Design review of the part built by this model. Coordinates are the model's own, in mm. A direction names the side the tool comes from. Coordinates: 2 decimals unless noted, no trailing zeros. Loops run counter-clockwise (first coordinate to the right, second up) from the corner with the lowest first, then second, coordinate; pieces in that order, holes last. Notation, with made-up numbers: (-1, -17.5) -> (35, -17.5) arc R33 ccw to (35, 21.5) -> close; hole circle Ø10 at (73, -33.75). An arc over 180 degrees is marked (long way). Answer as a JSON object with one key per item and string values.
```python
from build123d import *

# Parameters (mm, degrees)
F0_W     = 114
F0_H     = 100
F1_DEPTH = 2.4
F2_DEPTH = 52.4
F3_R     = 1.75
F4_DEPTH = 2.401
F5_DEPTH = 116.401


with BuildPart() as f1:
    # F0 (on Top) → F1 (new body)
    with BuildSketch(Plane.XY):
        Rectangle(F0_W, F0_H)
        Polygon((-57, -50), (-57, 50), (-59.4, 50), (-59.4, -52.4), (59.4, -52.4), (59.4, 50), (57, 50), (57, -50), align=None)
    extrude(amount=F1_DEPTH)

    # F0 (on Top) → F2 (join)
    with BuildSketch(Plane.XY):
        Polygon((-57, -50), (-57, 50), (-59.4, 50), (-59.4, -52.4), (59.4, -52.4), (59.4, 50), (57, 50), (57, -50), align=None)
    extrude(amount=F2_DEPTH)

    # F3 (on face) → F4 (cut, through all)
    with BuildSketch(Plane(origin=(57, 0, 0), x_dir=(0, -1, 0), z_dir=(-1, 0, 0))):
        with Locations((-40, 39.9)):
            Circle(F3_R)
        with Locations((-40, 14.9)):
            Circle(F3_R)
    extrude(amount=-F4_DEPTH, mode=Mode.SUBTRACT)

    # F3 (on face) → F5 (cut, through all)
    with BuildSketch(Plane(origin=(57, 0, 0), x_dir=(0, -1, 0), z_dir=(-1, 0, 0))):
        with Locations((-40, 39.9)):
            Circle(F3_R)
        with Locations((-40, 14.9)):
            Circle(F3_R)
    extrude(amount=F5_DEPTH, mode=Mode.SUBTRACT)


solid = f1.part
```
1) Wall thickness on probe 1 along Z at (x, y) = (-58.2, 40); probe 2 along X at (y, z) = (-47, 18.5); probe 3 along Y at (x, z) = (10, 41.5): over which ranges is each line inside the solid? List them lowest first.
Completed:
{"probe 1": "0 to 13.15, 16.65 to 38.15, 41.65 to 52.4", "probe 2": "-59.4 to -57, 57 to 59.4", "probe 3": "-52.4 to -50"}
2) Add section A-A, the plane y = 40. Give the boundary of the cut face in (x, z).
Completed:
{"outline": "(-59.4, 0) -> (59.4, 0) -> (59.4, 13.15) -> (57, 13.15) -> (57, 2.4) -> (-57, 2.4) -> (-57, 13.15) -> (-59.4, 13.15) -> close; (-59.4, 16.65) -> (-57, 16.65) -> (-57, 38.15) -> (-59.4, 38.15) -> close; (-59.4, 41.65) -> (-57, 41.65) -> (-57, 52.4) -> (-59.4, 52.4) -> close; (57, 16.65) -> (59.4, 16.65) -> (59.4, 38.15) -> (57, 38.15) -> close; (57, 41.65) -> (59.4, 41.65) -> (59.4, 52.4) -> (57, 52.4) -> close"}
3) For faces 1 (the flat face through (-26.7, -50.3, 52.4)), 2 (the flat face through (-57, -1, 27)), list the 3-axis set-ups (+Z, -Z, +X, -X, +Y, -Y) from which the entire face can be reached by the end or side of a thin tool; tool diameter is ignored.
Completed:
{"face 1": "+Z, +X, -X, +Y, -Y", "face 2": "+Z, +Y"}
4) Clearance check with flat-ended pins moving along their axes: pin 1 Ø2 at (y, z) = (40, 39.9) entering from +X; pin 2 Ø1 at (x, z) = (-46, 37) entering from +Y; pin 3 Ø2 at (x, y) = (34, -10.5) entering from +Z. State where each tip first meets the part, or that it passes through.
Completed:
{"pin 1": "through", "pin 2": "y = -50", "pin 3": "z = 2.4"}
5) Add section D-D, the plane x = 13. Give the boundary of the cut face in (y, z), and give its area (3 significant figures).
Completed:
{"outline": "(-52.4, 0) -> (50, 0) -> (50, 2.4) -> (-50, 2.4) -> (-50, 52.4) -> (-52.4, 52.4) -> close", "area": "366 mm²"}
6) Add section B-B, the plane z = 39.9. Give the boundary of the cut face in (x, y).
Completed:
{"outline": "(-59.4, -52.4) -> (59.4, -52.4) -> (59.4, 38.25) -> (57, 38.25) -> (57, -50) -> (-57, -50) -> (-57, 38.25) -> (-59.4, 38.25) -> close; (-59.4, 41.75) -> (-57, 41.75) -> (-57, 50) -> (-59.4, 50) -> close; (57, 41.75) -> (59.4, 41.75) -> (59.4, 50) -> (57, 50) -> close"}
7) Add section C-C, the plane z = 18. Give the boundary of the cut face in (x, y), and give its area (3 significant figures).
Completed:
{"outline": "(-59.4, -52.4) -> (59.4, -52.4) -> (59.4, 50) -> (57, 50) -> (57, -50) -> (-57, -50) -> (-57, 50) -> (-59.4, 50) -> close", "area": "765 mm²"}
8) The part is to be moulded in two halves that separate along Y. For faces 3 (the cylindrical face through (-58.183, 38.383, 14.23)), 4 (the flat face through (27, 50, 1)), 5 (the flat face through (-1, 1, 2.4)), say which applies: pulls with the +Y half, pulls with the -Y half, needs draft (parallel to the pull), parting line crosses it, or undercut.
Completed:
{"face 3": "undercut", "face 4": "pulls with the +Y half", "face 5": "needs draft"}
